from build123d import *

# Parameters (mm, degrees)
SKETCH1_R           = 2
SKETCH1_R_2         = 1.5
SKETCH1_R_3         = 5
BOSS_EXTRUDE1_DEPTH = 3


with BuildPart() as part:
    # Sketch1 → Boss-Extrude1 (new body)
    with BuildSketch(Plane.XY):
        with BuildLine():
            Line((-75, 50), (75, 50))
            ThreePointArc((75, 50), (82.071067812, 47.071067812), (85, 40))
            Line((85, 40), (85, -40))
            ThreePointArc((85, -40), (82.071067812, -47.071067812), (75, -50))
            Line((75, -50), (-75, -50))
            ThreePointArc((-75, -50), (-82.071067812, -47.071067812), (-85, -40))
            Line((-85, -40), (-85, 40))
            ThreePointArc((-85, 40), (-82.071067812, 47.071067812), (-75, 50))
        make_face()
        with Locations((-70.5, 8)):
            Circle(SKETCH1_R, mode=Mode.SUBTRACT)
        with Locations((-70.5, -8)):
            Circle(SKETCH1_R, mode=Mode.SUBTRACT)
        with Locations((-56.5, -8)):
            Circle(SKETCH1_R, mode=Mode.SUBTRACT)
        with Locations((-56.5, 8)):
            Circle(SKETCH1_R, mode=Mode.SUBTRACT)
        with Locations((70.5, -8)):
            Circle(SKETCH1_R, mode=Mode.SUBTRACT)
        with Locations((56.5, -8)):
            Circle(SKETCH1_R, mode=Mode.SUBTRACT)
        with Locations((56.5, 8)):
            Circle(SKETCH1_R, mode=Mode.SUBTRACT)
        with Locations((70.5, 8)):
            Circle(SKETCH1_R, mode=Mode.SUBTRACT)
        with Locations((-75, -40)):
            Circle(SKETCH1_R_2, mode=Mode.SUBTRACT)
        with Locations((-75, 40)):
            Circle(SKETCH1_R_2, mode=Mode.SUBTRACT)
        with Locations((75, 40)):
            Circle(SKETCH1_R_2, mode=Mode.SUBTRACT)
        with Locations((75, -40)):
            Circle(SKETCH1_R_2, mode=Mode.SUBTRACT)
        with Locations((-63.5, 0)):
            Circle(SKETCH1_R_3, mode=Mode.SUBTRACT)
        with Locations((63.5, 0)):
            Circle(SKETCH1_R_3, mode=Mode.SUBTRACT)
        with BuildLine():
            Line((-25, 45), (25, 45))
            ThreePointArc((25, 45), (30, 40), (25, 35))
            Line((25, 35), (-25, 35))
            ThreePointArc((-25, 35), (-30, 40), (-25, 45))
        make_face(mode=Mode.SUBTRACT)
        with BuildLine():
            Line((-25, -45), (25, -45))
            ThreePointArc((25, -45), (30, -40), (25, -35))
            Line((25, -35), (-25, -35))
            ThreePointArc((-25, -35), (-30, -40), (-25, -45))
        make_face(mode=Mode.SUBTRACT)
        with BuildLine():
            Line((-24, -27.5), (-24, -22.5))
            ThreePointArc((-24, -22.5), (-22.5, -21), (-21, -22.5))
            Line((-21, -22.5), (-21, -27.5))
            ThreePointArc((-21, -27.5), (-22.5, -29), (-24, -27.5))
        make_face(mode=Mode.SUBTRACT)
        with BuildLine():
            Line((-24, 27.5), (-24, 22.5))
            ThreePointArc((-24, 22.5), (-22.5, 21), (-21, 22.5))
            Line((-21, 22.5), (-21, 27.5))
            ThreePointArc((-21, 27.5), (-22.5, 29), (-24, 27.5))
        make_face(mode=Mode.SUBTRACT)
        with BuildLine():
            Line((24, 27.5), (24, 22.5))
            ThreePointArc((24, 22.5), (22.5, 21), (21, 22.5))
            Line((21, 22.5), (21, 27.5))
            ThreePointArc((21, 27.5), (22.5, 29), (24, 27.5))
        make_face(mode=Mode.SUBTRACT)
        with BuildLine():
            Line((24, -27.5), (24, -22.5))
            ThreePointArc((24, -22.5), (22.5, -21), (21, -22.5))
            Line((21, -22.5), (21, -27.5))
            ThreePointArc((21, -27.5), (22.5, -29), (24, -27.5))
        make_face(mode=Mode.SUBTRACT)
    extrude(amount=BOSS_EXTRUDE1_DEPTH)


solid = part.part
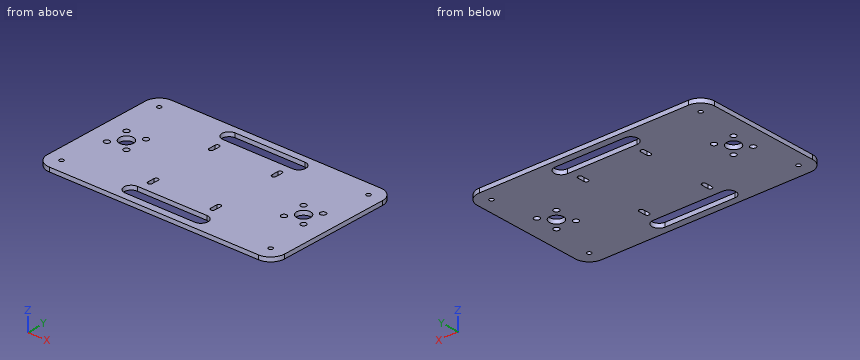
Can you work these out from the model? Positions are in its coordinate system, mm. Coordinates: 2 decimals unless noted, no trailing zeros. Write each loop counter-clockwise with the first axis right and the second up, starting at its lowest first coordinate (ties: lowest second). Pieces come first, ordered by that corner, then holes. Notation, with made-up numbers: (-37.5, -5.75) -> (-3.5, -5.75) arc R25 cw to (-3.5, 27.25) -> close; hole circle Ø1 at (68.25, -1.5). An arc over 180 degrees is marked (long way). Answer as CSV lines item,"result".
1) If we section it at B-B on y = 0: Please give me the cut outline in (x, z).
Check result:
outline,"(-85, 0) -> (-68.5, 0) -> (-68.5, 3) -> (-85, 3) -> close; (-58.5, 0) -> (58.5, 0) -> (58.5, 3) -> (-58.5, 3) -> close; (68.5, 0) -> (85, 0) -> (85, 3) -> (68.5, 3) -> close"
2) If we section it at C-C on x = -63.5: Please give me the cut outline in (y, z).
Check result:
outline,"(-50, 0) -> (-5, 0) -> (-5, 3) -> (-50, 3) -> close; (5, 0) -> (50, 0) -> (50, 3) -> (5, 3) -> close"
3) If we section it at D-D on z = 0.6: Count the separate pieces of the cut face and the enclosed holes in it, then the cut area to 3 significant figures.
Check result:
separate pieces,"1"
enclosed holes,"20"
area,"15,400 mm²"
4) If I drill on line 1 (Y direction, x = 56.5, z = 1.9); line 2 (Y direction, x = 7.5, z = 2.7); line 3 (X direction, y = 26, z = 1.95), over which ranges is the centre line in solid material (lowest first)? Write a range as from..to.
Check result:
line 1,"-50..-10, -6..6, 10..50"
line 2,"-50..-45, -35..35, 45..50"
line 3,"-85..-24, -21..21, 24..85"
5) If we section it at A-A on x = -9.5: Please give me the cut outline in (y, z), then the cut area to 3 significant figures.
Check result:
outline,"(-50, 0) -> (-45, 0) -> (-45, 3) -> (-50, 3) -> close; (-35, 0) -> (35, 0) -> (35, 3) -> (-35, 3) -> close; (45, 0) -> (50, 0) -> (50, 3) -> (45, 3) -> close"
area,"240 mm²"
